Check sheet for the modelled part. Datum: model origin and axes. Units: mm. Round coordinates to 2 decimals unless told otherwise and drop trailing zeros. Order: outer loops, then holes, each group sorted by start corner. A loop starts at its lowest first (then second) coordinate and runs counter-clockwise, first axis right, second up. Notation, with made-up numbers: (45.25, 59.25) -> (63.25, 59.25) arc R23 cw to (63.25, 96.25) -> close; hole circle Ø9 at (2.5, 88.25). An arc over 180 degrees is marked (long way). Answer in a Markdown table with one row per item. Add a question column.
1. Material ranges on L1, parallel to Y at x = 25.75, z = 39.95; L2, parallel to Z at x = 37.25, y = 141.4; L3, parallel to X at y = 142.45, z = 40, recorded low to high. Write a range as from..to.
2. Sectioned sample at A-A, the plane x = 15.5. Record the boundary of the cut face in (y, z), then the cut area to 3 significant figures.
3. Draft check along Z on faces 1 (the flat face through (40.44, 143, 39)), 2 (the flat face through (26, 143, 40.294)), 3 (the flat face through (26, 143, 37.294)). Enter one of: +Z half, -Z half, draft (parallel to the pull), parting line (faces both ways), or undercut.
```python
from build123d import *

# Parameters (mm, degrees)
BOSS_EXTRUDE1_START = 11.440071
SKETCH2_W           = 3
SKETCH2_H           = 3
BOSS_EXTRUDE1_DEPTH = 29
FILLET1_R           = 0.5
FILLET3_R           = 0.5


with BuildPart() as part:
    # Sketch2 → Boss-Extrude1 (new body)
    with BuildSketch(Plane(origin=(0, 0, 0), x_dir=(0, 0, -1), z_dir=(1, 0, 0)).offset(BOSS_EXTRUDE1_START)):
        with Locations((-38.793556796, 142.574028513)):
            Rectangle(SKETCH2_W, SKETCH2_H)
    extrude(amount=BOSS_EXTRUDE1_DEPTH)

    # Fillet1
    fillet1_edges = [part.edges().sort_by_distance(p)[0] for p in [
        (25.940071, 144.074028513, 40.293556796),
        (25.940071, 144.074028513, 37.293556796),
        (25.940071, 141.074028513, 37.293556796),
        (25.940071, 141.074028513, 40.293556796),
    ]]
    fillet(fillet1_edges, radius=FILLET1_R)

    # Fillet3
    fillet3_edges = [part.edges().sort_by_distance(p)[0] for p in [
        (40.440071, 144.074028513, 38.793556796),
        (11.440071, 144.074028513, 38.793556796),
        (11.440071, 142.574028513, 40.293556796),
        (11.440071, 142.574028513, 37.293556796),
        (11.440071, 141.074028513, 38.793556796),
        (11.440071, 141.220475122, 40.147110187),
        (11.440071, 141.220475122, 37.440003406),
        (11.440071, 143.927581903, 40.147110187),
        (11.440071, 143.927581903, 37.440003406),
        (40.440071, 142.574028513, 37.293556796),
        (40.440071, 141.074028513, 38.793556796),
        (40.440071, 142.574028513, 40.293556796),
        (40.440071, 141.220475122, 40.147110187),
        (40.440071, 141.220475122, 37.440003406),
        (40.440071, 143.927581903, 40.147110187),
        (40.440071, 143.927581903, 37.440003406),
    ]]
    fillet(fillet3_edges, radius=FILLET3_R)


solid = part.part
```
Answer key:
| question | item | result |
|---|---|---|
| 1 | L1 | y = 141.1..144.05 |
| 1 | L2 | z = 37.32..40.26 |
| 1 | L3 | x = 11.48..40.4 |
| 2 | outline | (141.07, 37.79) arc R0.5 ccw to (141.57, 37.29) -> (143.57, 37.29) arc R0.5 ccw to (144.07, 37.79) -> (144.07, 39.79) arc R0.5 ccw to (143.57, 40.29) -> (141.57, 40.29) arc R0.5 ccw to (141.07, 39.79) -> close |
| 2 | area | 8.79 mm² |
| 3 | face 1 | draft |
| 3 | face 2 | +Z half |
| 3 | face 3 | -Z half |
